The listing builds one solid part. Answer for the finished solid, in the listing's coordinates (mm). Face numbers are marked on the shaded views. Give positions to 0.01 mm unless a question says otherwise; leave off trailing zeros. Write each loop counter-clockwise with the first axis right and the second up, starting at its lowest first coordinate (ties: lowest second). Pieces come first, ordered by that corner, then holes.
Autodesk Inventor part; units mm, degrees
ref_plane "Work Plane1" through (0, 2.5, 0) normal (0, -1, 0) x (1, 0, 0)
ref_plane "YZ Plane" through (0, 0, 0) normal (1, 0, 0) x (0, 1, 0)
ref_plane "XZ Plane" through (0, 0, 0) normal (0, 1, 0) x (-1, 0, 0)
sketch "Sketch1" plane through (0, 0, 0) normal (0, 1, 0) x (-1, 0, 0)
  line L0 (0, 0) -> (59, 0)
  line L1 (59, 0) -> (59, -82)
  line L2 (59, -82) -> (0, -82)
  line L3 (0, -82) -> (0, 0)
  dimension "d0" = 82
  dimension "d1" = 59
extrude "Extrusion1" add sketch "Sketch1" along normal blind 32
ref_plane "Work Plane1" through (0, 2.5, 0) normal (0, -1, 0) x (1, 0, 0)
sketch "Sketch2" plane through (0, 2.5, 0) normal (0, -1, 0) x (1, 0, 0)
  line L0 (-2.5, -2.5) -> (-56.5, -2.5)
  line L1 (-56.5, -2.5) -> (-56.5, -79.5)
  line L2 (-56.5, -79.5) -> (-2.5, -79.5)
  line L3 (-2.5, -79.5) -> (-2.5, -2.5)
  line L4 (0, 0) -> (0, -82)
  line L5 (-59, 0) -> (0, 0)
  line L6 (-59, -82) -> (-59, 0)
  line L7 (0, -82) -> (-59, -82)
  dimension "d5" = 2.5
  dimension "d6" = 2.5
  dimension "d7" = 2.5
  dimension "d8" = 2.5
extrude "Extrusion2" cut sketch "Sketch2" against normal blind 27 contours L3 L2 L1 L0
sketch "Sketch3" plane through (0, 2.5, 0) normal (0, -1, 0) x (1, 0, 0)
  line L0 (-3, -3) -> (-56, -3) construction
  line L1 (-56, -3) -> (-56, -79) construction
  line L2 (-56, -79) -> (-3, -79) construction
  line L3 (-3, -79) -> (-3, -3) construction
  line L4 (-2.5, -2.5) -> (-2.5, -79.5)
  line L5 (-56.5, -2.5) -> (-2.5, -2.5)
  line L6 (-56.5, -79.5) -> (-56.5, -2.5)
  line L7 (-2.5, -79.5) -> (-56.5, -79.5)
  circle A0 centre (-53.8, -24.59) radius 1.65
  circle A1 centre (-5.54, -23.32) radius 1.65
  circle A2 centre (-38.56, -75.39) radius 1.65
  circle A3 centre (-10.62, -75.39) radius 1.65
  point P0 (0, 0)
  dimension "d11" = 0.5
  dimension "d12" = 0.5
  dimension "d13" = 0.5
  dimension "d14" = 0.5
  dimension "d15" = 3.3
  dimension "d16" = 20.32
  dimension "d17" = 2.54
  dimension "d18" = 7.62
  dimension "d19" = 72.39
  dimension "d20" = 21.59
  dimension "d22" = 50.8
  dimension "d23" = 35.56
  dimension "d24" = 72.39
extrude "Extrusion3" cut sketch "Sketch3" along normal blind 27 contours A0 | A1 | A2 | A3
sketch "Sketch4" plane through (-59, 0, 0) normal (0, 0, 1) x (1, 0, 0)
  line L0 (13.4, 5.6) -> (26.4, 5.6)
  line L1 (26.4, 5.6) -> (26.4, 16.5)
  line L2 (26.4, 16.5) -> (13.4, 16.5)
  line L3 (13.4, 16.5) -> (13.4, 5.6)
  line L4 (43.3, 5.6) -> (53.2, 5.6)
  line L5 (53.2, 5.6) -> (53.2, 16.5)
  line L6 (53.2, 16.5) -> (43.3, 16.5)
  line L7 (43.3, 16.5) -> (43.3, 5.6)
  line L8 (56.5, 2.5) -> (2.5, 2.5)
  line L9 (2.5, 2.5) -> (2.5, 29.5)
  line L10 (56.5, 2.5) -> (56.5, 29.5)
  point P0 (59, 0)
  dimension "d27" = 13
  dimension "d28" = 10.9
  dimension "d29" = 9.9
  dimension "d31" = 14
  dimension "d32" = 10.9
  dimension "d33" = 3.3
extrude "Extrusion4" cut sketch "Sketch4" against normal blind 5
sketch "Sketch5" plane through (0, 0, -82) normal (0, 0, -1) x (-1, 0, 0)
  line L0 (11.5, 24.5) -> (33.5, 24.5)
  line L1 (33.5, 24.5) -> (33.5, 20.5)
  line L2 (33.5, 20.5) -> (11.5, 20.5)
  line L3 (11.5, 20.5) -> (11.5, 24.5)
  line L4 (37.5, 24.5) -> (43.5, 24.5)
  line L5 (43.5, 24.5) -> (43.5, 20.5)
  line L6 (43.5, 20.5) -> (37.5, 20.5)
  line L7 (37.5, 20.5) -> (37.5, 24.5)
  line L8 (56.5, 2.5) -> (2.5, 2.5)
  line L9 (2.5, 2.5) -> (2.5, 29.5)
  point P0 (0, 0)
  dimension "d36" = 22
  dimension "d37" = 4
  dimension "d38" = 4
  dimension "d39" = 22
  dimension "d40" = 9
  dimension "d41" = 6
  dimension "d42" = 4
extrude "Extrusion5" cut sketch "Sketch5" against normal blind 5
sketch "Sketch6" plane through (-59, 0, -82) normal (-1, 0, 0) x (0, 0, 1)
  circle A0 centre (57.41, 6) radius 1.6
  line L0 (79.5, 2.5) -> (79.5, 29.5)
  line L1 (82, 0) -> (0, 0)
  dimension "d45" = 3.2
  dimension "d46" = 22.09
  dimension "d47" = 6
sketch "Sketch7" plane through (0, 0, 0) normal (1, 0, 0) x (0, 0, -1)
  circle A0 centre (23.32, 6) radius 1.6
  line L0 (82, 0) -> (0, 0)
  line L1 (2.5, 2.5) -> (2.5, 29.5)
  dimension "d48" = 6
  dimension "d49" = 20.82
  dimension "d50" = 3.2
sketch "Sketch8" plane through (0, 0, -82) normal (0, 0, -1) x (-1, 0, 0)
  circle A0 centre (10.62, 6) radius 1.6
  circle A1 centre (38.56, 6) radius 1.6
  line L0 (59, 0) -> (0, 0)
  line L1 (2.5, 2.5) -> (2.5, 29.5)
  dimension "d51" = 3.2
  dimension "d52" = 3.2
  dimension "d53" = 6
  dimension "d54" = 6
  dimension "d55" = 8.12
  dimension "d56" = 36.06
extrude "Extrusion6" cut sketch "Sketch6" against normal blind 5
extrude "Extrusion7" cut sketch "Sketch7" against normal blind 5
extrude "Extrusion8" cut sketch "Sketch8" against normal blind 5
sketch "Sketch9" plane through (-59, 0, 0) normal (0, 0, 1) x (1, 0, 0)
  line L0 (-2.1645, 16) -> (66.4826, 16)
  line L1 (59, 0) -> (0, 0)
  dimension "d63" = 16
properties part number "Arduino_Box"
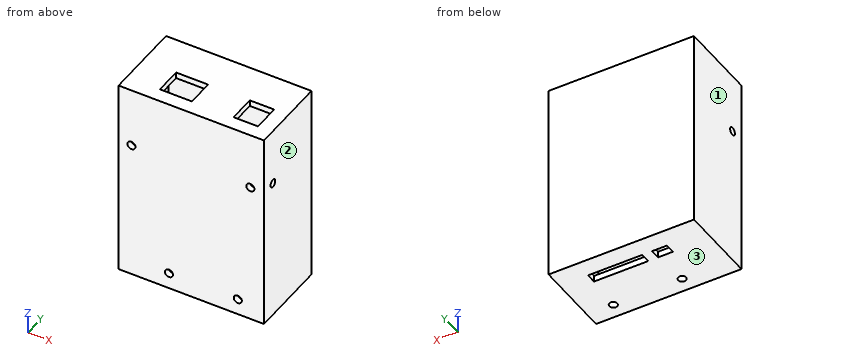
Item 1: A cutting plane is placed at A-A, the plane z = -75.39. Give the vertices of the cut face in (x, y).
Conclusion:
outline: (-59, 0) - (-40.21, 0) - (-40.21, 2.5) - (-56.5, 2.5) - (-56.5, 29.5) - (-2.5, 29.5) - (-2.5, 2.5) - (-8.97, 2.5) - (-8.97, 0) - (0, 0) - (0, 32) - (-59, 32) - close; (-36.91, 0) - (-12.27, 0) - (-12.27, 2.5) - (-36.91, 2.5) - close
Item 2: A cutting plane is placed at C-C, the plane x = -38.56. Give the vertices of the cut face in (y, z).
Conclusion:
outline: (0, -82) - (4.4, -82) - (4.4, -79.5) - (2.5, -79.5) - (2.5, -77.04) - (0, -77.04) - close; (0, -73.74) - (2.5, -73.74) - (2.5, -2.5) - (5.6, -2.5) - (5.6, 0) - (0, 0) - close; (7.6, -82) - (20.5, -82) - (20.5, -79.5) - (7.6, -79.5) - close; (16.5, -2.5) - (29.5, -2.5) - (29.5, -79.5) - (24.5, -79.5) - (24.5, -82) - (32, -82) - (32, 0) - (16.5, 0) - close
Item 3: A cutting plane is placed at B-B, the plane y = 23.5. Give the vertices of the cut face in (x, z), plus the area to 3 significant figures.
Conclusion:
outline: (-59, -82) - (-43.5, -82) - (-43.5, -79.5) - (-56.5, -79.5) - (-56.5, -2.5) - (-2.5, -2.5) - (-2.5, -79.5) - (-11.5, -79.5) - (-11.5, -82) - (0, -82) - (0, 0) - (-59, 0) - close; (-37.5, -82) - (-33.5, -82) - (-33.5, -79.5) - (-37.5, -79.5) - close
area: 610 mm2
Item 4: This flat-tipped pin is pushed along its axis until it touches: P1, Ø3, axis at x = -53.8, z = -24.59, coming from the -Y side. Where does it stop, or does it pass through?
Conclusion:
P1: stops at y = 29.5
Item 5: Consider probe 1 along X at (y, z) = (1.05, -75.39); probe 2 along X at (y, z) = (13.5, -51); probe 3 along Y at (x, z) = (-21, -77.5). Determine where each line is inside the solid, lowest interval first.
Conclusion:
probe 1: x = -59 to -40.21, -36.91 to -12.27, -8.97 to 0
probe 2: x = -59 to -56.5, -2.5 to 0
probe 3: y = 0 to 2.5, 29.5 to 32
Item 6: Determine the mould class of the marked faces 1, 2 and 3 for opening direction X: pulls with the +X half, pulls with the -X half, needs draft (parallel to the pull), parting line crosses it, or undercut.
Conclusion:
face 1: pulls with the -X half
face 2: pulls with the +X half
face 3: needs draft
Item 7: A cutting plane is placed at D-D, the plane z = -50.5. Give the vertices of the cut face in (x, y).
Conclusion:
outline: (-59, 0) - (0, 0) - (0, 32) - (-59, 32) - close; hole (-56.5, 2.5) - (-2.5, 2.5) - (-2.5, 29.5) - (-56.5, 29.5) - close
